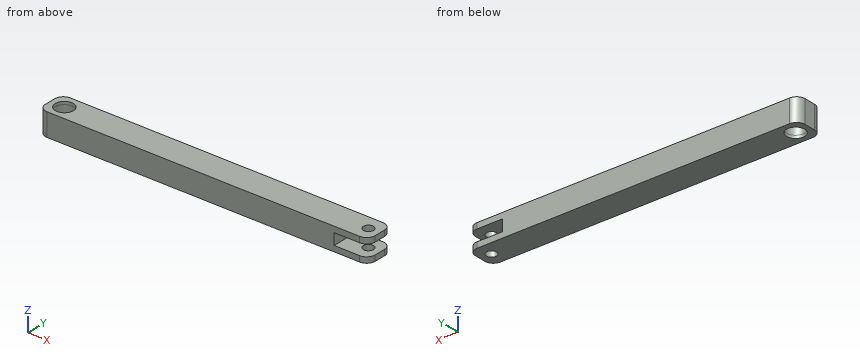
```python
from build123d import *

# Parameters (mm, degrees)
SKETCH_5_W          = 58
SKETCH_5_H          = 3
EXTRUDE_1_DEPTH     = 5
CUT_EXTRUDE_1_REACH = 60.292
SKETCH_6_R          = 1.6
CUT_EXTRUDE_2_REACH = 60.292
SKETCH_7_R          = 0.9
FILLET_1_R          = 1.5
SKETCH_8_W          = 6
SKETCH_8_H          = 1.6
CUT_EXTRUDE_3_DEPTH = 10
SKETCH_10_R         = 1.6
SKETCH_10_R_2       = 0.9
EXTRUDE_2_DEPTH     = 0.5
EXTRUDE_START       = 0.5
SKETCH_11_R         = 0.9
SKETCH_11_R_2       = 1.6
EXTRUDE_3_DEPTH     = 0.5
SKETCH_12_W         = 6.44666191
SKETCH_12_H         = 2
CUT_EXTRUDE_4_DEPTH = 10


with BuildPart() as part:
    # 草图5 → 凸台-拉伸1 (new body)
    with BuildSketch(Plane(origin=(0, 0, 0), x_dir=(1, 0, 0), z_dir=(0, 1, 0))):
        with Locations((29, -1.5)):
            Rectangle(SKETCH_5_W, SKETCH_5_H)
    extrude(amount=EXTRUDE_1_DEPTH)

    # 草图6 → 切除-拉伸1 (cut, up to next)
    with BuildSketch(Plane.XY.offset(3), mode=Mode.PRIVATE) as cut_extrude_1_sk1:
        with Locations((2.5, 2.5)):
            Circle(SKETCH_6_R)
    cut_extrude_1_tool1 = extrude(cut_extrude_1_sk1.sketch, amount=-CUT_EXTRUDE_1_REACH, mode=Mode.PRIVATE) & part.part
    add(cut_extrude_1_tool1.solids().sort_by_distance((2.5, 2.5, 3))[0], mode=Mode.SUBTRACT)

    # 草图7 → 切除-拉伸2 (cut, up to next)
    with BuildSketch(Plane.XY, mode=Mode.PRIVATE) as cut_extrude_2_sk1:
        with Locations(Location((56, 2.5, 0), (0, 0, 180))):
            Circle(SKETCH_7_R)
    cut_extrude_2_tool1 = extrude(cut_extrude_2_sk1.sketch, amount=CUT_EXTRUDE_2_REACH, mode=Mode.PRIVATE) & part.part
    add(cut_extrude_2_tool1.solids().sort_by_distance((56, 2.5, 0))[0], mode=Mode.SUBTRACT)

    # 圆角1
    fillet_1_edges = [part.edges().sort_by_distance(p)[0] for p in [
        (58, 5, 1.5),
        (58, 0, 1.5),
        (0, 0, 1.5),
        (0, 5, 1.5),
    ]]
    fillet(fillet_1_edges, radius=FILLET_1_R)

    # 草图8 → 切除-拉伸3 (cut)
    with BuildSketch(Plane(origin=(0, 5, 0), x_dir=(1, 0, 0), z_dir=(0, 1, 0))):
        with Locations((55, -1.5)):
            Rectangle(SKETCH_8_W, SKETCH_8_H)
    extrude(amount=-CUT_EXTRUDE_3_DEPTH, mode=Mode.SUBTRACT)

    # 草图10 → 凸台-拉伸2 (add)
    with BuildSketch(Plane.XY.offset(3)):
        with BuildLine():
            Line((58, 1.5), (58, 3.5))
            ThreePointArc((58, 3.5), (57.560660172, 4.560660172), (56.5, 5))
            Line((56.5, 5), (1.5, 5))
            ThreePointArc((1.5, 5), (0.439339828, 4.560660172), (0, 3.5))
            Line((0, 3.5), (0, 1.5))
            ThreePointArc((0, 1.5), (0.439339828, 0.439339828), (1.5, 0))
            Line((1.5, 0), (56.5, 0))
            ThreePointArc((56.5, 0), (57.560660172, 0.439339828), (58, 1.5))
        make_face()
        with Locations((2.5, 2.5)):
            Circle(SKETCH_10_R, mode=Mode.SUBTRACT)
        with Locations(Location((56, 2.5, 0), (0, 0, 180))):
            Circle(SKETCH_10_R_2, mode=Mode.SUBTRACT)
    extrude(amount=EXTRUDE_2_DEPTH)

    # 草图11 → 凸台-拉伸3 (add)
    with BuildSketch(Plane(origin=(0, 0, 0), x_dir=(-1, 0, 0), z_dir=(0, 0, -1)).offset(EXTRUDE_START)):
        with BuildLine():
            Line((-1.5, 5), (-56.5, 5))
            ThreePointArc((-56.5, 5), (-57.560660172, 4.560660172), (-58, 3.5))
            Line((-58, 3.5), (-58, 1.5))
            ThreePointArc((-58, 1.5), (-57.560660172, 0.439339828), (-56.5, 0))
            Line((-56.5, 0), (-1.5, 0))
            ThreePointArc((-1.5, 0), (-0.439339828, 0.439339828), (0, 1.5))
            Line((0, 1.5), (0, 3.5))
            ThreePointArc((0, 3.5), (-0.439339828, 4.560660172), (-1.5, 5))
        make_face()
        with Locations((-56, 2.5)):
            Circle(SKETCH_11_R, mode=Mode.SUBTRACT)
        with Locations(Location((-2.5, 2.5, 0), (0, 0, 180))):
            Circle(SKETCH_11_R_2, mode=Mode.SUBTRACT)
    extrude(amount=-EXTRUDE_3_DEPTH)

    # 草图12 → 切除-拉伸4 (cut)
    with BuildSketch(Plane.XZ):
        with Locations((55.223330955, 1.5)):
            Rectangle(SKETCH_12_W, SKETCH_12_H)
    extrude(amount=-CUT_EXTRUDE_4_DEPTH, mode=Mode.SUBTRACT)


solid = part.part
```
Here's how the part is built. I have some questions about the finished solid (model axes, mm). Round coordinates to 2 decimals unless told otherwise and drop trailing zeros. Order: outer loops, then holes, each group sorted by start corner. A loop starts at its lowest first (then second) coordinate and runs counter-clockwise, first axis right, second up. Notation, with made-up numbers: M -27.75,73 L -9.75,73 A21 cw -9.75,83 Z; hole C 82,61 d4. An arc over 180 degrees is marked long. One line per question, with ' | ' between items.
1) I want a section at A-A, the plane y = 2.5. Write out the boundary of the cut face in (x, z), then the cut area to 3 significant figures.
Working result:
outline: M 0,-0.5 L 0.9,-0.5 L 0.9,3.5 L 0,3.5 Z; M 4.1,-0.5 L 55.1,-0.5 L 55.1,0.5 L 52,0.5 L 52,2.5 L 55.1,2.5 L 55.1,3.5 L 4.1,3.5 Z; M 56.9,-0.5 L 58,-0.5 L 58,0.5 L 56.9,0.5 Z; M 56.9,2.5 L 58,2.5 L 58,3.5 L 56.9,3.5 Z | area: 204 mm²
2) For pin 1 Ø1.6 at (x, y) = (56, 2.5) entering from +Z; pin 2 Ø1.5 at (y, z) = (0.5, 1.5) entering from -X, each with a flat end and sliding along its axis, tell me the tip position at first contact or that it passes through.
Working result:
pin 1: through | pin 2: x = 0.02
3) I want a section at B-B, the plane x = 56. Write out the boundary of the cut face in (y, z), then the cut area to 3 significant figures.
Working result:
outline: M 0,-0.5 L 1.6,-0.5 L 1.6,0.5 L 0,0.5 Z; M 0,2.5 L 1.6,2.5 L 1.6,3.5 L 0,3.5 Z; M 3.4,-0.5 L 5,-0.5 L 5,0.5 L 3.4,0.5 Z; M 3.4,2.5 L 5,2.5 L 5,3.5 L 3.4,3.5 Z | area: 6.40 mm²
4) I need wall thicknesses on line 1 along Y through (x, z) = (2.5, 3.15); line 2 along X through (y, z) = (2.6, 1.6); line 3 along X through (y, z) = (1.9, 1.5). Which ranges of each line are inside material? Lowest first, please.
Working result:
line 1: 0 to 0.9, 4.1 to 5 | line 2: 0 to 0.9, 4.1 to 52 | line 3: 0 to 1.02, 3.98 to 52
5) I want a section at D-D, the plane x = 2.5. Write out the boundary of the cut face in (y, z).
Working result:
outline: M 0,-0.5 L 0.9,-0.5 L 0.9,3.5 L 0,3.5 Z; M 4.1,-0.5 L 5,-0.5 L 5,3.5 L 4.1,3.5 Z
6) I want a section at C-C, the plane z = 1.35. Write out the boundary of the cut face in (x, y).
Working result:
outline: M 0,1.5 A1.5 ccw 1.5,0 L 52,0 L 52,5 L 1.5,5 A1.5 ccw 0,3.5 Z; hole C 2.5,2.5 d3.2
